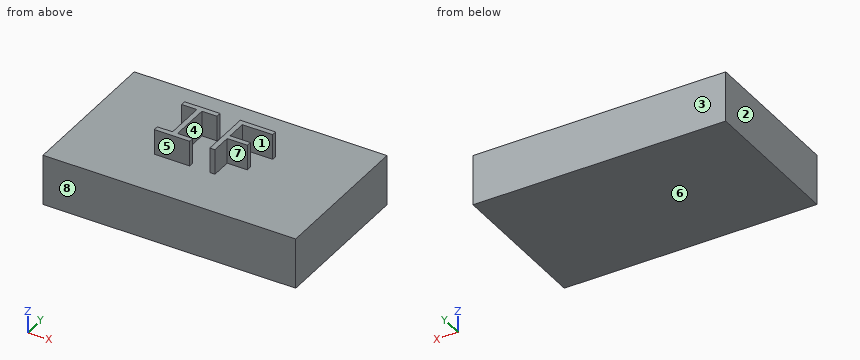
Autodesk Inventor part; units mm, degrees
ref_plane "YZ Plane" through (0, 0, 0) normal (1, 0, 0) x (0, 1, 0)
ref_plane "XZ Plane" through (0, 0, 0) normal (0, 1, 0) x (-1, 0, 0)
ref_plane "XY Plane" through (0, 0, 0) normal (0, 0, 1) x (1, 0, 0)
sketch "Sketch1" plane through (0, 0, 0) normal (0, 0, 1) x (1, 0, 0)
  line L0 (0, 0) -> (50, 0)
  line L1 (50, 0) -> (50, 30)
  line L2 (50, 30) -> (0, 30)
  line L3 (0, 30) -> (0, 0)
  dimension "d0" = 50
  dimension "d1" = 30
extrude "Extrusion1" add sketch "Sketch1" along normal blind 10
sketch "Sketch2" plane through (0, 0, 10) normal (0, 0, 1) x (1, 0, 0)
  line L0 (0, 0) -> (50, 0)
  line L1 (50, 30) -> (0, 30)
  line L2 (0, 0) -> (50, 0)
  line L3 (50, 0) -> (50, 30)
  line L4 (50, 30) -> (0, 30)
  line L5 (0, 30) -> (0, 0)
  line L6 (16, 20) -> (23, 20)
  line L7 (23, 20) -> (23, 19)
  line L8 (23, 19) -> (20, 19)
  line L9 (20, 19) -> (20, 11)
  line L10 (20, 11) -> (23, 11)
  line L11 (23, 11) -> (23, 10)
  line L12 (23, 10) -> (16, 10)
  line L13 (16, 10) -> (16, 11)
  line L14 (16, 11) -> (19, 11)
  line L15 (19, 11) -> (19, 19)
  line L16 (19, 19) -> (16, 19)
  line L17 (16, 19) -> (16, 20)
  line L18 (27, 10) -> (27, 20)
  line L19 (27, 20) -> (34, 20)
  line L20 (34, 20) -> (34, 19)
  line L21 (34, 19) -> (28, 19)
  line L22 (28, 19) -> (28, 15)
  line L23 (28, 15) -> (32, 15)
  line L24 (32, 15) -> (32, 14)
  line L25 (32, 14) -> (28, 14)
  line L26 (28, 14) -> (28, 10)
  line L27 (28, 10) -> (27, 10)
  point P0 (17.5, 19)
  point P1 (16, 10.5)
  point P2 (23, 10.5)
  point P3 (23, 19.5)
  point P4 (31, 19)
  point P5 (30, 14)
  point P6 (27, 15)
  dimension "d4" = 1
  dimension "d5" = 1
  dimension "d6" = 1
  dimension "d7" = 3
  dimension "d8" = 3
  dimension "d9" = 10
  dimension "d10" = 10
  dimension "d11" = 30
  dimension "d12" = 50
  dimension "d13" = 23
  dimension "d14" = 23
  dimension "d15" = 10
  dimension "d16" = 1
  dimension "d17" = 1
  dimension "d18" = 1
  dimension "d19" = 7
  dimension "d20" = 4
  dimension "d21" = 10
  dimension "d22" = 4
extrude "Extrusion2" add sketch "Sketch2" along normal blind 5 contours L6 L7 L8 L9 L10 L11 L12 L13 L14 L15 L16 L17 | L18 L19 L20 L21 L22 L23 L24 L25 L26 L27
equation "\"d6\" = d5"
equation "\"d10\" = -0.5 * d9 + 0.5 * d11"
equation "\"d14\" = d13"
equation "\"d15\" = d10"
equation "\"d19\" = d8 + d7 + d5"
equation "\"d20\" = d7 + d5"
equation "\"d21\" = d9"
equation "\"d22\" = -0.5 * d17 + 0.5 * d21 - 0.5 * d16"
properties part number "Names"
Verification items for the finished model (mm, model axes). Face numbers are marked on the shaded views. A direction names the side the tool comes from. Round coordinates to 2 decimals unless told otherwise and drop trailing zeros. Write each loop counter-clockwise with the first axis right and the second up, starting at its lowest first coordinate (ties: lowest second). Pieces come first, ordered by that corner, then holes. Notation, with made-up numbers: (-22.5, 23.5) -> (4.5, 23.5) arc R15 ccw to (4.5, 43.5) -> close; hole circle Ø5 at (19.5, -34.5). An arc over 180 degrees is marked (long way). Write each question's results on one line, items separated by ' | '. Start each with the question number.
1. Depth check by flat-ended pin: P1, Ø0.5, axis at y = 19.5, z = 12, coming from the +X side; P2, Ø1, axis at x = 7.5, y = 25.5, coming from the +Z side; P3, Ø0.5, axis at y = 10.5, z = 11.5, coming from the -X side. Enter the tip coordinate at first touch or a pass-through.
2. Cross-section at C-C (y = 25). Enter the section's corners in (x, z), then the cut area to 3 significant figures.
3. Draft check along Y on the marked faces 1, 2 and 3. Enter one of: +Y half, -Y half, draft (parallel to the pull), parting line (faces both ways), or undercut.
4. Cross-section at D-D (x = 42). Enter the section's corners in (y, z), then the cut area to 3 significant figures.
5. Material ranges on probe 1 along Y at (x, z) = (30, 13); probe 2 along X at (y, z) = (18.5, 13.5); probe 3 along Z at (x, y) = (46.5, 12.25), recorded low to high. Write a range as from..to.
6. Set-up check for the marked faces 4, 5, 6, 7 and 8: record each of +Z, -Z, +X, -X, +Y, -Y from which the full face is reachable in a straight line by a thin tool's end or side.
7. Cross-section at B-B (x = 33). Enter the section's corners in (y, z), then the cut area to 3 significant figures.
8. Cross-section at A-A (z = 14). Enter the section's corners in (x, y), then the cut area to 3 significant figures.
Solutions:
1) P1: stops at x = 34 | P2: stops at z = 10 | P3: stops at x = 16
2) outline: (0, 0) -> (50, 0) -> (50, 10) -> (0, 10) -> close | area: 500 mm2
3) face 1: undercut | face 2: draft | face 3: +Y half
4) outline: (0, 0) -> (30, 0) -> (30, 10) -> (0, 10) -> close | area: 300 mm2
5) probe 1: y = 14..15, 19..20 | probe 2: x = 19..20, 27..28 | probe 3: z = 0..10
6) face 4: +Z | face 5: +Z, +X, -X, -Y | face 6: -Z, +X, -X, +Y, -Y | face 7: +Z, +X, -Y | face 8: +Z, -Z, +X, -X, -Y
7) outline: (0, 0) -> (30, 0) -> (30, 10) -> (20, 10) -> (20, 15) -> (19, 15) -> (19, 10) -> (0, 10) -> close | area: 305 mm2
8) outline: (16, 10) -> (23, 10) -> (23, 11) -> (20, 11) -> (20, 19) -> (23, 19) -> (23, 20) -> (16, 20) -> (16, 19) -> (19, 19) -> (19, 11) -> (16, 11) -> close; (27, 10) -> (28, 10) -> (28, 14) -> (32, 14) -> (32, 15) -> (28, 15) -> (28, 19) -> (34, 19) -> (34, 20) -> (27, 20) -> close | area: 42.0 mm2
